Could you check a few things on this model? Use its own coordinates, in mm. Face numbers are marked on the shaded views. A direction names the side the tool comes from. Coordinates: 2 decimals unless noted, no trailing zeros. Loops run counter-clockwise (first coordinate to the right, second up) from the corner with the lowest first, then second, coordinate; pieces in that order, holes last.
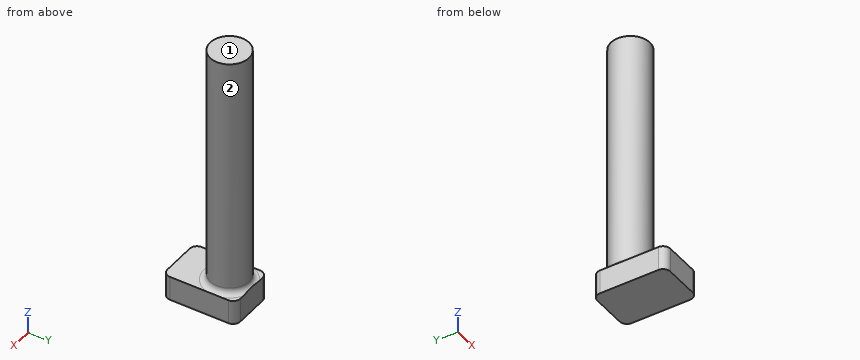
Autodesk Inventor part; units mm, degrees
ref_plane "YZ Plane" through (0, 0, 0) normal (1, 0, 0) x (0, 1, 0)
ref_plane "XZ Plane" through (0, 0, 0) normal (0, 1, 0) x (-1, 0, 0)
ref_plane "XY Plane" through (0, 0, 0) normal (0, 0, 1) x (1, 0, 0)
sketch "スケッチ1" plane through (0, 0, 0) normal (0, 0, 1) x (1, 0, 0)
  line L0 (5, 7.5) -> (-5, 7.5)
  line L1 (-5, 7.5) -> (-5, -7.5)
  line L2 (-5, -7.5) -> (5, -7.5)
  line L3 (5, -7.5) -> (5, 7.5)
  line L4 (5, 7.5) -> (-5, -7.5) construction
  line L5 (-5, 7.5) -> (5, -7.5) construction
  point P0 (0, 0)
  dimension "d0" = 10
  dimension "d1" = 15
extrude "押し出し1" add sketch "スケッチ1" along normal blind 5
sketch "スケッチ2" plane through (0, 0, 5) normal (0, 0, 1) x (1, 0, 0)
  line L0 (0, 0) -> (0, 3)
  circle A0 centre (0, 3) radius 4
  dimension "d4" = 3
  dimension "d5" = 8
extrude "押し出し2" add sketch "スケッチ2" along normal blind 50
fillet "フィレット1" radius 1.2 1 edges at (-4, 3, 5)
fillet "フィレット2" radius 1.5 4 edges at (5, 7.5, 2.5) (-5, 7.5, 2.5) (5, -7.5, 2.5) (-5, -7.5, 2.5)
properties part number "slidev"
(1) Imagine slicing it at B-B, the plane x = 0. Write out the boundary of the cut face in (y, z).
Answers:
outline: (-7.5, 0) - (7.5, 0) - (7.5, 5.23) arc R1.2 cw to (7, 6.2) - (7, 55) - (-1, 55) - (-1, 6.2) arc R1.2 cw to (-2.2, 5) - (-7.5, 5) - close
(2) Imagine slicing it at C-C, the plane z = 10. Write out the boundary of the cut face in (x, y).
Answers:
outline: circle Ø8 at (0, 3)
(3) For pin 1 (3 mm diameter, centred on x = -2, z = 25, fed in from -Y); pin 2 (1.5 mm diameter, centred on y = 0.5, z = 21, fed in from +X); pin 3 (2 mm diameter, centred on y = -1, z = 16.5, fed in from +X); pin 4 (2.5 mm diameter, centred on x = -0.5, y = -1, fed in from +Z), each with a flat end and sliding along its axis, tell me the tip position at first contact or that it passes through.
Answers:
pin 1: stops at y = -0.97
pin 2: stops at x = 3.6
pin 3: stops at x = 2.65
pin 4: stops at z = 55
(4) Which directions (+Z, -Z, +X, -X, +Y, -Y) give clear straight access to the entire face, cutting with the end or side of a thin tool? Please do the marked faces 1 and 2.
Answers:
face 1: +Z, +X, -X, +Y, -Y
face 2: +Z
(5) Imagine slicing it at A-A, the plane y = 3. Write out the boundary of the cut face in (x, z), and give its area (3 significant figures).
Answers:
outline: (-5, 0) - (5, 0) - (5, 5.02) arc R1.2 cw to (4, 6.2) - (4, 55) - (-4, 55) - (-4, 6.2) arc R1.2 cw to (-5, 5.02) - close
area: 451 mm2
(6) I need wall thicknesses on probe 1 along Y at (x, z) = (0.25, 51); probe 2 along Z at (x, y) = (4.5, -3.5); probe 3 along Y at (x, z) = (-3.5, 52.5). Which ranges of each line are inside material? Lowest first, please.
Answers:
probe 1: y = -0.99 to 6.99
probe 2: z = 0 to 5
probe 3: y = 1.06 to 4.94
